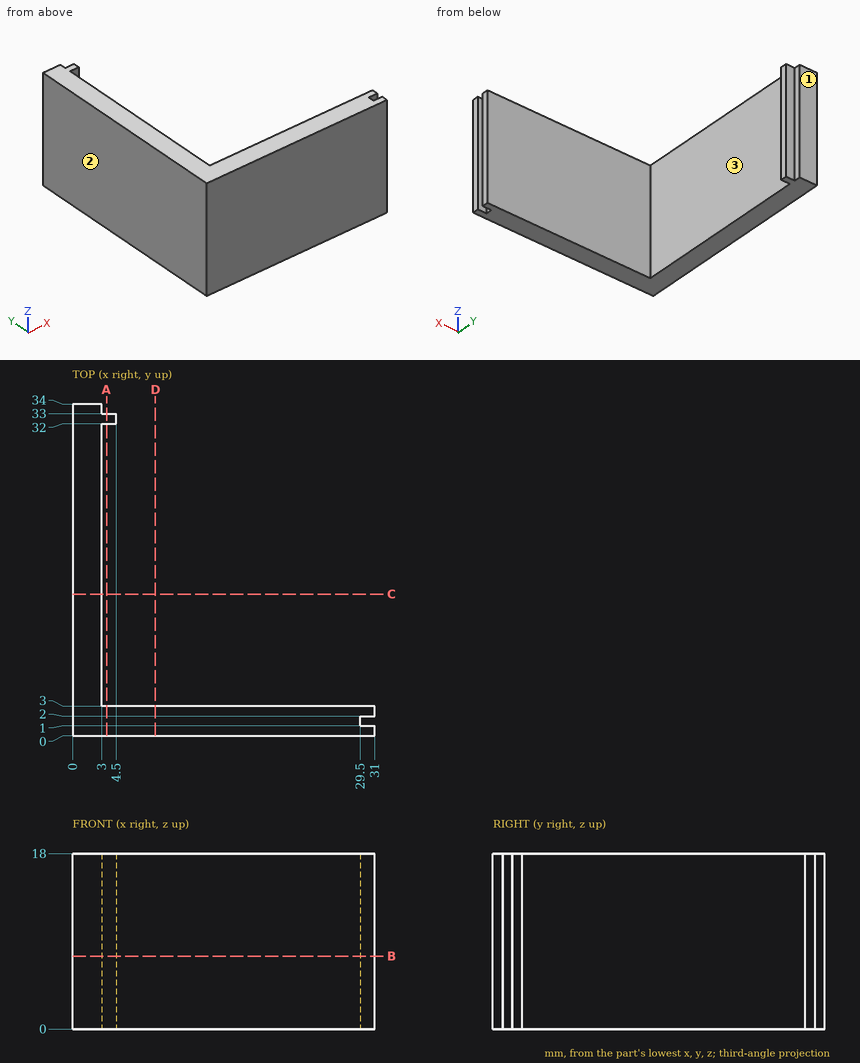
The figure shows three views and two pictorial views of one solid part (mm, origin at its lowest corner). Answer the questions. Coordinates: 2 decimals unless noted, no trailing zeros. Write each loop counter-clockwise with the first axis right and the second up, starting at its lowest first coordinate (ties: lowest second). Pieces come first, ordered by that corner, then holes. Notation, with made-up numbers: (75, -39.75) -> (84, -39.75) arc R29 cw to (84, -8.75) -> close; hole circle Ø8 at (30, 82). An arc over 180 degrees is marked (long way). Return JSON: item names as keys, results as strings.
(1) Consider line 1 along Y through (x, z) = (4, 2.25); line 2 along Y through (x, z) = (7, 10.5). Determine where each line is inside the solid, lowest interval first. Write a range as from..to.
Answers below:
{"line 1": "0..3, 32..33", "line 2": "0..3"}
(2) The part is cut by section B-B on z = 7.5. Give the vertices of the cut face in (x, y).
Answers below:
{"outline": "(0, 0) -> (31, 0) -> (31, 1) -> (29.5, 1) -> (29.5, 2) -> (31, 2) -> (31, 3) -> (3, 3) -> (3, 32) -> (4.5, 32) -> (4.5, 33) -> (3, 33) -> (3, 34) -> (0, 34) -> close"}
(3) The part is cut by section A-A on x = 3.5. Give the vertices of the cut face in (y, z), then the cut area to 3 significant figures.
Answers below:
{"outline": "(0, 0) -> (3, 0) -> (3, 18) -> (0, 18) -> close; (32, 0) -> (33, 0) -> (33, 18) -> (32, 18) -> close", "area": "72.0 mm^2"}
(4) For a pull along Y with two mould halves and no side action, classify the marked faces 1, 2 and 3 as pulls with the +Y half, pulls with the -Y half, needs draft (parallel to the pull), parting line crosses it, or undercut.
Answers below:
{"face 1": "pulls with the +Y half", "face 2": "needs draft", "face 3": "undercut"}
(5) The part is cut by section C-C on y = 14.5. Give the vertices of the cut face in (x, z).
Answers below:
{"outline": "(0, 0) -> (3, 0) -> (3, 18) -> (0, 18) -> close"}
(6) Each of these flat-tipped pins is pushed along its axis until it touches: P1, Ø1.2, axis at x = 4, z = 7.5, coming from the +Y side; P2, Ø10, axis at x = 12.5, z = 14.5, coming from the -Y side; P3, Ø5, axis at y = 27, z = 15, coming from the +X side; P4, Ø0.8, axis at y = 1.5, z = 6, coming from the +X side. Where does it stop, or does it pass through?
Answers below:
{"P1": "y = 33", "P2": "y = 0", "P3": "x = 3", "P4": "x = 29.5"}
